Verification items for the finished model (mm, model axes). A direction names the side the tool comes from. Give positions to 0.01 mm unless a question says otherwise; leave off trailing zeros. Write each loop counter-clockwise with the first axis right and the second up, starting at its lowest first coordinate (ties: lowest second). Pieces come first, ordered by that corner, then holes. Notation, with made-up numbers: M 45.5,-35 L 88.5,-35 A19 ccw 88.5,-8 Z; hole C 66,78.25 d10. An arc over 180 degrees is marked long. Answer as a JSON object with one key per item and string values.
```python
from build123d import *

# Parameters (mm, degrees)
ESQUISSE1_R        = 1.6
BOSS_EXTRU_1_DEPTH = 15


with BuildPart() as part:
    # Esquisse1 → Boss.-Extru.1 (new body)
    with BuildSketch(Plane(origin=(0, 0, 0), x_dir=(1, 0, 0), z_dir=(0, 1, 0))):
        with BuildLine():
            Line((0.379867182, -77.5), (4, -77.5))
            ThreePointArc((4, -77.5), (5.224744871, -77.08113883), (5.936491673, -76))
            ThreePointArc((5.936491673, -76), (5.224744871, -74.91886117), (4, -74.5))
            Line((4, -74.5), (2, -74.5))
            ThreePointArc((2, -74.5), (0.585786438, -73.914213562), (0, -72.5))
            Line((0, -72.5), (0, -72))
            ThreePointArc((0, -72), (-14.427005158, -37.9049997), (-0.571883425, -3.573627385))
            ThreePointArc((-0.571883425, -3.573627385), (-0.148482629, -2.929684622), (0, -2.173454879))
            Line((0, -2.173454879), (0, 0))
            ThreePointArc((0, 0), (-0.585786438, 1.414213562), (-2, 2))
            Line((-2, 2), (-20.553034366, 2))
            ThreePointArc((-20.553034366, 2), (-21.847406556, 1.524664105), (-22.526517183, 0.324600632))
            ThreePointArc((-22.526517183, 0.324600632), (-22.651920818, -0.115392313), (-22.874034374, -0.515374102))
            ThreePointArc((-22.874034374, -0.515374102), (-30.332217892, -44.419762154), (-0.360571251, -77.357888836))
            ThreePointArc((-0.360571251, -77.357888836), (0.002890838, -77.46415092), (0.379867182, -77.5))
        make_face()
        with Locations(Location((-17.168486885, -2.5, 0), (0, 0, 90))):
            Circle(ESQUISSE1_R, mode=Mode.SUBTRACT)
        with BuildLine():
            Line((-26.245903328, -16.4), (-11.593054617, -16.4))
            ThreePointArc((-11.593054617, -16.4), (-10.579787815, -16.103547862), (-11.273476907, -16.899405215))
            ThreePointArc((-11.273476907, -16.899405215), (-13.352037133, -22.277466593), (-14.794641856, -27.85983602))
            ThreePointArc((-14.794641856, -27.85983602), (-14.547802836, -28.823941756), (-15.448193173, -28.4))
            Line((-15.448193173, -28.4), (-28.185804557, -28.4))
            ThreePointArc((-28.185804557, -28.4), (-29.132721919, -28.780731674), (-28.712919494, -27.850476321))
            ThreePointArc((-28.712919494, -27.850476321), (-28.139109588, -22.339660076), (-26.947329323, -16.928743953))
            ThreePointArc((-26.947329323, -16.928743953), (-27.126974093, -15.960805113), (-26.245903328, -16.4))
        make_face(mode=Mode.SUBTRACT)
        with BuildLine():
            Line((-28.216882659, -29.9), (-15.703506193, -29.9))
            ThreePointArc((-15.703506193, -29.9), (-14.736948258, -29.540862859), (-15.234489879, -30.444005186))
            ThreePointArc((-15.234489879, -30.444005186), (-15.668556704, -34.886741932), (-15.702797946, -39.350501707))
            ThreePointArc((-15.702797946, -39.350501707), (-15.282185488, -40.280514324), (-16.229311222, -39.9))
            Line((-16.229311222, -39.9), (-27.241766652, -39.9))
            ThreePointArc((-27.241766652, -39.9), (-28.141135688, -40.3247838), (-27.897916749, -39.360340703))
            ThreePointArc((-27.897916749, -39.360340703), (-28.536105971, -34.925039157), (-28.766778335, -30.44999999))
            ThreePointArc((-28.766778335, -30.44999999), (-29.155828271, -29.511128156), (-28.216882659, -29.9))
        make_face(mode=Mode.SUBTRACT)
        with BuildLine():
            Line((-14.218448274, -51.7), (-23.236538966, -51.7))
            ThreePointArc((-23.236538966, -51.7), (-24.079106647, -52.165729699), (-24.025281338, -51.204518335))
            ThreePointArc((-24.025281338, -51.204518335), (-25.860949004, -46.797976835), (-27.259486048, -42.233836401))
            ThreePointArc((-27.259486048, -42.233836401), (-27.825028416, -41.361102537), (-26.841844264, -41.7))
            Line((-26.841844264, -41.7), (-16.109676342, -41.7))
            ThreePointArc((-16.109676342, -41.7), (-15.188659613, -41.293986962), (-15.510234208, -42.247773197))
            ThreePointArc((-15.510234208, -42.247773197), (-14.870347536, -46.748469382), (-13.822458806, -51.172003072))
            ThreePointArc((-13.822458806, -51.172003072), (-13.228444983, -52.029995612), (-14.218448274, -51.7))
        make_face(mode=Mode.SUBTRACT)
        with BuildLine():
            Line((-22.201450768, -53.7), (-13.576816642, -53.7))
            ThreePointArc((-13.576816642, -53.7), (-12.708653375, -53.251366369), (-12.844917969, -54.219049971))
            ThreePointArc((-12.844917969, -54.219049971), (-11.418475339, -57.778687264), (-9.722191927, -61.217928288))
            ThreePointArc((-9.722191927, -61.217928288), (-8.984061268, -61.980064854), (-10.007414918, -61.7))
            Line((-10.007414918, -61.7), (-16.734180973, -61.7))
            ThreePointArc((-16.734180973, -61.7), (-17.517935865, -62.197854045), (-17.635485157, -61.276815206))
            ThreePointArc((-17.635485157, -61.276815206), (-20.215891111, -57.835366348), (-22.484800972, -54.181038342))
            ThreePointArc((-22.484800972, -54.181038342), (-23.225348113, -53.420856119), (-22.201450768, -53.7))
        make_face(mode=Mode.SUBTRACT)
        with BuildLine():
            Line((-14.676144728, -64), (-8.645402719, -64))
            ThreePointArc((-8.645402719, -64), (-7.830810759, -63.517826697), (-7.799980557, -64.463924289))
            ThreePointArc((-7.799980557, -64.463924289), (-4.628127789, -68.842617177), (-1, -72.851393816))
            Line((-1, -72.851393816), (-1, -74.351393816))
            ThreePointArc((-1, -74.351393816), (-8.358263561, -69.980068178), (-14.84445078, -64.395992083))
            ThreePointArc((-14.84445078, -64.395992083), (-15.7323224, -63.784862453), (-14.676144728, -64))
        make_face(mode=Mode.SUBTRACT)
        with BuildLine():
            Line((-3.068400716, -4.1), (-12.868400716, -4.1))
            ThreePointArc((-12.868400716, -4.1), (-14.468400716, -2.5), (-12.868400716, -0.9))
            Line((-12.868400716, -0.9), (-3.068400716, -0.9))
            ThreePointArc((-3.068400716, -0.9), (-1.468400716, -2.5), (-3.068400716, -4.1))
        make_face(mode=Mode.SUBTRACT)
        with BuildLine():
            Line((-11.011595694, -15.2), (-25.878211235, -15.2))
            ThreePointArc((-25.878211235, -15.2), (-26.873424632, -15.52293193), (-26.257429531, -14.677186831))
            ThreePointArc((-26.257429531, -14.677186831), (-24.539239864, -10.245004819), (-22.4, -6))
            Line((-22.4, -6), (-4.5, -6))
            ThreePointArc((-4.5, -6), (-7.584699304, -10.204982732), (-10.212442966, -14.709670602))
            ThreePointArc((-10.212442966, -14.709670602), (-10.173962247, -15.668793132), (-11.011595694, -15.2))
        make_face(mode=Mode.SUBTRACT)
    extrude(amount=-BOSS_EXTRU_1_DEPTH)


solid = part.part
```
1) Section check B-B on x = -6.5. Record the boundary of the cut face in (y, z), and give its area (3 significant figures).
Completed:
{"outline": "M -15,-2 L 0,-2 L 0,0.9 L -15,0.9 Z; M -15,4.1 L 0,4.1 L 0,6 L -15,6 Z; M -15,8.62 L 0,8.62 L 0,10.94 L -15,10.94 Z; M -15,64.06 L 0,64.06 L 0,66.38 L -15,66.38 Z; M -15,71.25 L 0,71.25 L 0,74.42 L -15,74.42 Z", "area": "189 mm2"}
2) Section check A-A on z = 57.5. Record the boundary of the cut face in (x, y), and give its area (3 significant figures).
Completed:
{"outline": "M -24.38,-15 L -20.44,-15 L -20.44,0 L -24.38,0 Z; M -11.54,-15 L -10.11,-15 L -10.11,0 L -11.54,0 Z", "area": "80.6 mm2"}
3) Section check D-D on y = -3.5. Count the separate pieces of the cut face and the enclosed holes in it, and give its area (3 significant figures).
Completed:
{"separate pieces": "1", "enclosed holes": "8", "area": "615 mm2"}
4) Release check for a two-part mould opening along X. For faces 1 (the face through (-12, -7, 64)), 2 (the face through (5.2, -7.4, 77.1)), 3 (the face through (-15, 0, 35)) record: pulls with the +X half, pulls with the -X half, needs draft (parallel to the pull), parting line crosses it, or undercut.
Completed:
{"face 1": "undercut", "face 2": "pulls with the +X half", "face 3": "needs draft"}
5) Thickness scan on L1, parallel to Z at x = -5, y = -11.75; L2, parallel to X at y = -3, z = 16; L3, parallel to Z at x = -19, y = -1.5. Record the ranges inside material, lowest first.
Completed:
{"L1": "z = -2 to 0.9, 4.1 to 6, 6.62 to 8.78, 66.22 to 68.38, 72.19 to 75.23", "L2": "x = -30.38 to -27.17, -26.42 to -11.42, -10.67 to -9.4", "L3": "z = -2 to 6, 15.2 to 16.4, 28.4 to 29.9, 39.9 to 41.7, 51.7 to 53.7, 59.54 to 64.5"}
6) Access from +Z, -Z, +X, -X, +Y, -Y to the whole of each face (thin tool, end or side, straight path). Record for faces 4 (the face through (-0.153, -7.395, 2.94)), 5 (the face through (2, -7, 77.5)), 6 (the face through (-25.84, -7.4, 46.86)).
Completed:
{"face 4": "+X, +Y, -Y", "face 5": "+Z, +X, -X, +Y, -Y", "face 6": "+Y, -Y"}
7) Section check C-C on z = 11. Record the boundary of the cut face in (x, y), and give its area (3 significant figures).
Completed:
{"outline": "M -28.65,-15 L -24.87,-15 L -24.87,0 L -28.65,0 Z; M -8.1,-15 L -6.54,-15 L -6.54,0 L -8.1,0 Z", "area": "80.1 mm2"}
8) Go/stop test with flat-tipped pins: pin 1 (3 mm diameter, centred on x = -22.5, y = -13.5, fed in from +Z); pin 2 (1.6 mm diameter, centred on y = -10, z = 73.5, fed in from -X); pin 3 (1.9 mm diameter, centred on x = -17.17, z = 2.5, fed in from +Y); pin 4 (5 mm diameter, centred on x = -9, y = -6, fed in from +Z). Record where each tip stops, or that it passes through.
Completed:
{"pin 1": "stops at z = 62.19", "pin 2": "stops at x = -9.33", "pin 3": "passes through", "pin 4": "stops at z = 74.42"}
